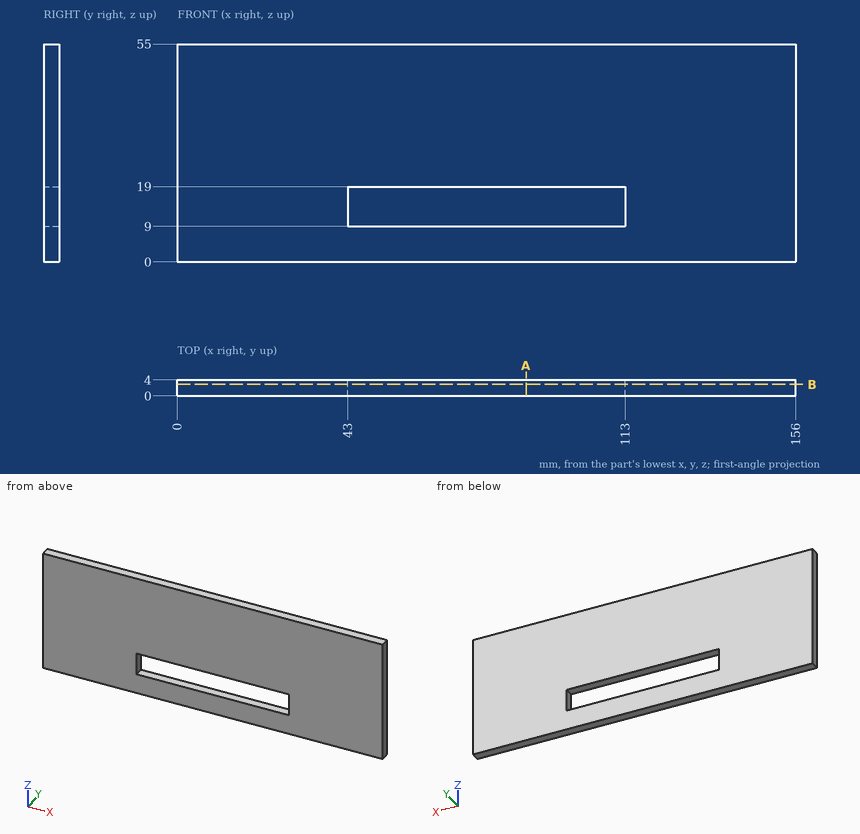
Verification items for this drawing (mm, ordinates from the low corner). Coordinates: 2 decimals unless noted, no trailing zeros. Write each loop counter-clockwise with the first axis right and the second up, starting at its lowest first coordinate (ties: lowest second). Pieces come first, ordered by that corner, then holes. Notation, with made-up numbers: (42.5, -26) -> (82.5, -26) arc R24 ccw to (82.5, 1) -> close; hole circle Ø5 at (34, 15.5). An arc over 180 degrees is marked (long way). Use CSV: the item, a comma, the result in double quotes. Start each with the question number.
Item 1: Depth check by flat-ended pin: pin 1 Ø2 at (x, y) = (76, 2) entering from -Z. Enter the tip coordinate at first touch or a pass-through.
Item 2: Cross-section at A-A, the plane x = 88. Record the cut outline in (y, z), plus the area to 3 significant figures.
Item 3: Cross-section at B-B, the plane y = 2.85. Record the cut outline in (x, z), plus the area to 3 significant figures.
Item 4: Thickness scan on line 1 (Z direction, x = 84.5, y = 1.35); line 2 (X direction, y = 3, z = 11.5). Record the ranges inside material, lowest first.
Answers:
1,pin 1,"z = 0"
2,outline,"(0, 0) -> (4, 0) -> (4, 9) -> (0, 9) -> close; (0, 19) -> (4, 19) -> (4, 55) -> (0, 55) -> close"
2,area,"180 mm^2"
3,outline,"(0, 0) -> (156, 0) -> (156, 55) -> (0, 55) -> close; hole (43, 9) -> (113, 9) -> (113, 19) -> (43, 19) -> close"
3,area,"7,880 mm^2"
4,line 1,"0 to 9, 19 to 55"
4,line 2,"0 to 43, 113 to 156"
